Source: CAD feature listing. Evaluate the final solid. Frame: model axes, mm. Round coordinates to 2 decimals unless told otherwise and drop trailing zeros. Order: outer loops, then holes, each group sorted by start corner. A loop starts at its lowest first (then second) coordinate and runs counter-clockwise, first axis right, second up. Notation, with made-up numbers: (-37, 47) - (6, 47) arc R23 ccw to (6, 79) - close; hole circle Ø10 at (63, -31.75). An arc over 180 degrees is marked (long way). Put each result on its own line as item: value. Start each with the question number.
1) Contact query for flat-ended pins moving along their axis: P1, Ø7.5, axis at x = 16.28, y = -5.47, coming from the -Z side; P2, Ø3.5, axis at x = 16.28, y = 16.12, coming from the -Z side. Output: stop coordinate, or through.
2) Section C-C on x = 90.5. Output: boundary loops of the cut face in (y, z), then the cut area to 3 significant figures.
3) Section B-B on y = 2.5. Output: boundary loops of the cut face in (x, z).
4) Line query: probe 1 along X at (y, z) = (17, 0.65); probe 2 along X at (y, z) = (-7.5, 1.3); probe 3 along Y at (x, z) = (103.5, 1.25). Output: solid intervals per line, ascending. Write a range as [from, to].
5) Section A-A on z = 0.6. State how many separate pieces and enclosed holes the cut face has, then the cut area to 3 significant figures.
Autodesk Inventor part; units mm, degrees
ref_plane "YZ Plane" through (0, 0, 0) normal (1, 0, 0) x (0, 1, 0)
ref_plane "XZ Plane" through (0, 0, 0) normal (0, 1, 0) x (-1, 0, 0)
ref_plane "XY Plane" through (0, 0, 0) normal (0, 0, 1) x (1, 0, 0)
sketch "Sketch1" plane through (0, 0, 0) normal (0, 0, 1) x (1, 0, 0)
  arc A0 (79.7785, -14.0465) -> (84.541, -9.284) centre (79.7785, -9.284) ccw
  circle A1 centre (3.5785, -9.284) radius 2.0828
  circle A2 centre (79.7785, -9.284) radius 2.3114
  arc A3 (84.541, 16.116) -> (79.7785, 20.8785) centre (79.7785, 16.116) ccw
  line L0 (23.4149, 20.8785) -> (79.7785, 20.8785)
  line L1 (84.541, 16.116) -> (84.541, -9.284)
  line L2 (79.7785, -14.0465) -> (3.5785, -14.0465)
  arc A4 (3.4793, -14.0455) -> (3.5785, -14.0465) centre (3.5785, -9.284) ccw
  arc A5 (-0.8541, -7.5424) -> (3.5785, -14.0465) centre (3.5785, -9.284) ccw
  line L3 (-0.8541, -7.5424) -> (8.7305, 16.8507)
  line L4 (23.4149, 20.8785) -> (14.6406, 20.8785)
  arc A6 (14.6406, 20.8785) -> (8.7305, 16.8507) centre (14.6406, 14.5285) ccw
  circle A7 centre (79.7785, 16.116) radius 2.0955
  point P0 (0, 0)
  point P1 (3.4793, -14.0455)
  dimension "d1" = 4.6228
  dimension "d5" = 9.525
  dimension "d6" = 6.35
  dimension "d9" = 4.191
  dimension "d25" = 4.1656
extrude "Extrusion1" add sketch "Sketch1" along normal blind 1.5875 contours L2 A4 A5 L3 A6 L4 L0 A3 L1 A0 | A7
sketch "Sketch2" plane through (41.6785, -9.284, 1.5875) normal (0, 0, 1) x (1, 0, 0)
  arc A0 (42.8625, 25.4) -> (38.1, 30.1625) centre (38.1, 25.4) ccw
  circle A1 centre (63.5, 25.4) radius 2.3114
  arc A2 (66.8676, 22.0324) -> (63.5, 30.1625) centre (63.5, 25.4) ccw
  line L0 (38.1, 30.1625) -> (63.5, 30.1625)
  arc A3 (38.1, -4.7625) -> (42.8625, 0) centre (38.1, 0) ccw
  line L1 (38.1, 30.1625) -> (-27.0379, 30.1625)
  line L2 (38.1, 30.1625) -> (35.3924, 30.1625)
  arc A4 (38.1, -4.7625) -> (41.4676, -3.3676) centre (38.1, 0) ccw
  line L3 (41.4676, -3.3676) -> (38.1, 30.1625)
  circle A5 centre (-25.4, 25.4) radius 2.3114
  circle A6 centre (38.1, 0) radius 2.3114
  arc A7 (41.4676, -3.3676) -> (42.8625, 0) centre (38.1, 0) ccw
  arc A8 (63.5, 20.6375) -> (63.5, 30.1625) centre (63.5, 25.4) ccw
  arc A9 (63.5, 20.6375) -> (42.8625, 0) centre (63.5, 0) ccw
  circle A10 centre (-25.4, 3.81) radius 2.3114
  point P0 (-41.6785, 9.284)
  point P1 (66.8676, 22.0324)
  dimension "d15" = 9.525
  dimension "d18" = 4.6228
  dimension "d22" = 4.6228
  dimension "d24" = 4.6228
extrude "Extrusion3" add sketch "Sketch2" against normal blind 1.5875 contours A8 A9 A3 L3 L0 A2
extrude "Extrusion4" cut sketch "Sketch2" against normal blind 1.5875 contours A5 | A10
properties part number "intake_base_outer" material "Acetal Resin, White"
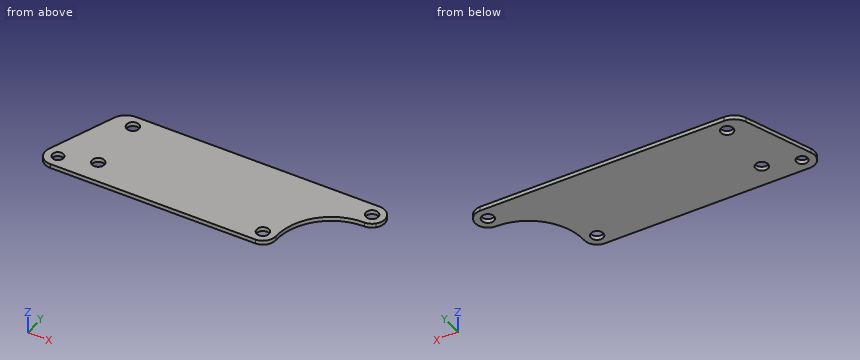
Answer sheet:
1. P1: z = 0
1. P2: through
2. outline: (5.22, 0) - (20.88, 0) - (20.88, 1.59) - (5.22, 1.59) - close
2. area: 24.9 mm^2
3. outline: (3.09, 0) - (88.24, 0) - (88.24, 1.59) - (3.09, 1.59) - close
4. probe 1: [8.79, 14.14], [18.41, 103.04], [107.31, 109.86]
4. probe 2: [-0.84, 2.5], [4.65, 15.17], [17.39, 78.31], [81.25, 84.62]
4. probe 3: [11.29, 14.53], [17.71, 20.88]
5. separate pieces: 1
5. enclosed holes: 5
5. area: 3,060 mm^2
